Could you check a few things on this model? Use its own coordinates, in mm. A direction names the side the tool comes from. Coordinates: 2 decimals unless noted, no trailing zeros. Loops run counter-clockwise (first coordinate to the right, second up) from the corner with the lowest first, then second, coordinate; pieces in that order, holes last. Notation, with made-up numbers: (42, 60) -> (94, 60) arc R21 cw to (94, 73) -> close; hole circle Ø1 at (48, 60). An arc over 180 degrees is marked (long way). One line per question, with ' | ' between items.
from build123d import *

# Parameters (mm, degrees)
CROQUIS1_R              = 2
SALIENTE_EXTRUIR1_DEPTH = 4


with BuildPart() as part:
    # Croquis1 → Saliente-Extruir1 (new body)
    with BuildSketch(Plane.XY):
        with BuildLine():
            ThreePointArc((57.381944444, -3.682723418), (59, 0), (57.381944444, 3.682723418))
            ThreePointArc((57.381944444, 3.682723418), (40.658639918, 40.658639918), (3.682723418, 57.381944444))
            ThreePointArc((3.682723418, 57.381944444), (0, 59), (-3.682723418, 57.381944444))
            ThreePointArc((-3.682723418, 57.381944444), (-40.658639918, 40.658639918), (-57.381944444, 3.682723418))
            ThreePointArc((-57.381944444, 3.682723418), (-59, 0), (-57.381944444, -3.682723418))
            ThreePointArc((-57.381944444, -3.682723418), (-40.658639918, -40.658639918), (-3.682723418, -57.381944444))
            ThreePointArc((-3.682723418, -57.381944444), (0, -59), (3.682723418, -57.381944444))
            ThreePointArc((3.682723418, -57.381944444), (40.658639918, -40.658639918), (57.381944444, -3.682723418))
        make_face()
        with BuildLine():
            ThreePointArc((-3.451039553, 50.381944444), (0, 49), (3.451039553, 50.381944444))
            ThreePointArc((3.451039553, 50.381944444), (35.70889245, 35.70889245), (50.381944444, 3.451039553))
            ThreePointArc((50.381944444, 3.451039553), (49, 0), (50.381944444, -3.451039553))
            ThreePointArc((50.381944444, -3.451039553), (35.70889245, -35.70889245), (3.451039553, -50.381944444))
            ThreePointArc((3.451039553, -50.381944444), (0, -49), (-3.451039553, -50.381944444))
            ThreePointArc((-3.451039553, -50.381944444), (-50.5, 0), (-3.451039553, 50.381944444))
        make_face(mode=Mode.SUBTRACT)
        with Locations((54, 0)):
            Circle(CROQUIS1_R, mode=Mode.SUBTRACT)
        with Locations((0, 54)):
            Circle(CROQUIS1_R, mode=Mode.SUBTRACT)
        with Locations((0, -54)):
            Circle(CROQUIS1_R, mode=Mode.SUBTRACT)
        with Locations((-54, 0)):
            Circle(CROQUIS1_R, mode=Mode.SUBTRACT)
    extrude(amount=SALIENTE_EXTRUIR1_DEPTH)


solid = part.part
1) If we section it at C-C on x = 13.5: Please give me the cut outline in (y, z), and give its area (3 significant figures).
Data:
outline: (-55.89, 0) -> (-48.66, 0) -> (-48.66, 4) -> (-55.89, 4) -> close; (48.66, 0) -> (55.89, 0) -> (55.89, 4) -> (48.66, 4) -> close | area: 57.8 mm²
2) I'm going to push a flat-ended pin straight in: pin 1 Ø2 at (x, z) = (-31.5, 3) entering from -Y. Where does the tip first touch, or does it pass through?
Data:
pin 1: y = -48.74
3) If we section it at D-D on x = 0: Please give me the cut outline in (y, z), and give its area (3 significant figures).
Data:
outline: (-59, 0) -> (-56, 0) -> (-56, 4) -> (-59, 4) -> close; (-52, 0) -> (-49, 0) -> (-49, 4) -> (-52, 4) -> close; (49, 0) -> (52, 0) -> (52, 4) -> (49, 4) -> close; (56, 0) -> (59, 0) -> (59, 4) -> (56, 4) -> close | area: 48.0 mm²
4) On a 3-axis mill with a long thin cutter (end or side, diameter ignored), from which of +Z, -Z, +X, -X, +Y, -Y can I reach the whole of each face in a straight line? I mean faces 1 (the face through (59, 0, 2)), 2 (the face through (0, -49, 2)). Say none if no direction works.
Data:
face 1: +Z, -Z, +X | face 2: +Z, -Z
5) If we section it at B-B on z = 1.5: Please give me the cut outline in (x, y).
Data:
outline: (-57.38, -3.68) arc R57.5 ccw to (-3.68, -57.38) arc R5 ccw to (3.68, -57.38) arc R57.5 ccw to (57.38, -3.68) arc R5 ccw to (57.38, 3.68) arc R57.5 ccw to (3.68, 57.38) arc R5 ccw to (-3.68, 57.38) arc R57.5 ccw to (-57.38, 3.68) arc R5 ccw to start; hole circle Ø4 at (-54, 0); hole (-3.45, -50.38) arc R5 cw to (3.45, -50.38) arc R50.5 ccw to (50.38, -3.45) arc R5 cw to (50.38, 3.45) arc R50.5 ccw to (3.45, 50.38) arc R5 cw to (-3.45, 50.38) arc R50.5 ccw to start; hole circle Ø4 at (0, -54); hole circle Ø4 at (0, 54); hole circle Ø4 at (54, 0)
6) I need wall thicknesses on line 1 along Y through (x, z) = (44.5, 3.15); line 2 along X through (y, z) = (-17, 2.7); line 3 along Y through (x, z) = (-33.5, 2.6). Which ranges of each line are inside material? Lowest first, please. Write a range as from..to.
Data:
line 1: -36.41..-23.87, 23.87..36.41 | line 2: -54.93..-47.55, 47.55..54.93 | line 3: -46.73..-37.79, 37.79..46.73
7) We'd pull the mould along X, two halves only. Please class faces 3 (the face through (49, 0, 2)), 4 (the face through (-41.067, -40.246, 1.972)), 5 (the face through (0, -59, 2)): pulls with the +X half, pulls with the -X half, needs draft (parallel to the pull), parting line crosses it, or undercut.
Data:
face 3: undercut | face 4: pulls with the -X half | face 5: parting line crosses it
8) If we section it at A-A on y = 0: Please give me the cut outline in (x, z).
Data:
outline: (-59, 0) -> (-56, 0) -> (-56, 4) -> (-59, 4) -> close; (-52, 0) -> (-50.5, 0) -> (-50.5, 4) -> (-52, 4) -> close; (49, 0) -> (52, 0) -> (52, 4) -> (49, 4) -> close; (56, 0) -> (59, 0) -> (59, 4) -> (56, 4) -> close
